Autodesk Inventor part; units mm, degrees
ref_plane "YZ Plane" through (0, 0, 0) normal (1, 0, 0) x (0, 1, 0)
ref_plane "XZ Plane" through (0, 0, 0) normal (0, 1, 0) x (-1, 0, 0)
ref_plane "XY Plane" through (0, 0, 0) normal (0, 0, 1) x (1, 0, 0)
sketch "Эскиз1" plane through (0, 0, 0) normal (0, 1, 0) x (-1, 0, 0)
  circle A0 centre (0, 0) radius 8.75
  dimension "d0" = 17.5
sketch "Эскиз2" plane through (0, 0, 0) normal (0, 1, 0) x (-1, 0, 0)
  circle A0 centre (0, 0) radius 12
  dimension "d1" = 24
extrude "Выдавливание1" add sketch "Эскиз2" along normal blind 1
extrude "Выдавливание2" add sketch "Эскиз1" against normal blind 4
sketch "Эскиз3" plane through (0, 1, 0) normal (0, 1, 0) x (1, 0, 0)
  circle A0 centre (0, 0) radius 8
  dimension "d6" = 16
extrude "Выдавливание3" cut sketch "Эскиз3" against normal blind 6
properties part number "Blumat_holder"
Read the model definition and answer for the solid it produces. Units are mm, in the model's axes. A direction names the side the tool comes from. Give positions to 0.01 mm unless a question says otherwise; leave off trailing zeros. Write each loop counter-clockwise with the first axis right and the second up, starting at its lowest first coordinate (ties: lowest second). Pieces come first, ordered by that corner, then holes. Notation, with made-up numbers: (70.5, 4) - (109.5, 4) arc R21 ccw to (109.5, 23) - close; hole circle Ø2 at (-40, 13.5). An arc over 180 degrees is marked (long way). Write item = value, one per line. Start each with the question number.
Item 1: Find section B-B (z = 0). Give the vertices of the cut face in (x, y), then the cut area to 3 significant figures.
Item 2: Find the intervals of material crossed by probe 1 along Z at (x, y) = (0, -1.05); probe 2 along Y at (x, z) = (-8, -4.5); probe 3 along Z at (x, y) = (0, 0.75), in increasing order. Write a range as [from, to].
Item 3: Find section C-C (z = 9.5). Give the vertices of the cut face in (x, y), then the cut area to 3 significant figures.
Item 4: Each of these flat-tipped pins is pushed along its axis until it touches: P1, Ø2, axis at y = -2.5, z = -6, coming from the -X side; P2, Ø1.5, axis at y = -2, z = -3.5, coming from the -X side; P3, Ø1, axis at y = 0, z = 1, coming from the -X side. Where does it stop, or does it pass through?
Item 5: Find section A-A (x = 0). Give the vertices of the cut face in (y, z), then the cut area to 3 significant figures.
Item 6: The mould has two halves that part along Z. Classify faces 3 (the flat face through (-2, 1, -8)), 4 (the cylindrical face through (-1.73, -1.46, 7.81)), 5 (the cylindrical face through (6.944, -1.972, -5.324)): +Z half, -Z half, draft (parallel to the pull), parting line (faces both ways), or undercut.
Item 7: A tool of negligible diameter and unlimited length cuts with its end or side. For faces 1 (the flat face through (-1, 0, -9)), 2 (the cylindrical face through (11.99, 0.49, -0.53)), from which of +Z, -Z, +X, -X, +Y, -Y can it reach the whole face along a straight path? Write none if from no direction.
Item 8: Find section D-D (x = -9.75). Give the vertices of the cut face in (y, z), then the cut area to 3 significant figures.
Response:
q1.outline = (-12, 0) - (-8.75, 0) - (-8.75, -4) - (-8, -4) - (-8, 1) - (-12, 1) - close; (8, -4) - (8.75, -4) - (8.75, 0) - (12, 0) - (12, 1) - (8, 1) - close
q1.area = 14.0 mm²
q2.probe_1 = [-8.75, -8], [8, 8.75]
q2.probe_2 = [0, 1]
q2.probe_3 = [-12, -8], [8, 12]
q3.outline = (-7.33, 0) - (7.33, 0) - (7.33, 1) - (-7.33, 1) - close
q3.area = 14.7 mm²
q4.P1 = -7.18
q4.P2 = -8.31
q4.P3 = -11.99
q5.outline = (-4, -8.75) - (0, -8.75) - (0, -12) - (1, -12) - (1, -8) - (-4, -8) - close; (-4, 8) - (1, 8) - (1, 12) - (0, 12) - (0, 8.75) - (-4, 8.75) - close
q5.area = 14.0 mm²
q6.face_3 = draft
q6.face_4 = undercut
q6.face_5 = parting line
q7.face_1 = -Y
q7.face_2 = +Y, -Y
q8.outline = (0, -7) - (1, -7) - (1, 7) - (0, 7) - close
q8.area = 14.0 mm²
